from build123d import *

# Parameters (mm, degrees)
F1_DEPTH = 12.7
F2_DEPTH = 17.78


with BuildPart() as f1:
    # F0 (on Front) → F1 (new body)
    with BuildSketch(Plane.XZ):
        with BuildLine():
            ThreePointArc((-7.62, 17.4596133978), (-3.8920987123, 18.6481652613), (0, 19.05))
            Line((0, 19.05), (0, 25.4309050116))
            ThreePointArc((0, 25.4309050116), (-1.335031029, 25.3955492468), (-2.6663651194, 25.2901575092))
            Line((-2.6663651194, 25.2901575092), (-2.6663651194, 22.86))
            Line((-2.6663651194, 22.86), (-4.8713176481, 22.86))
            Line((-4.8713176481, 22.86), (-4.8713176481, 24.9589173434))
            ThreePointArc((-4.8713176481, 24.9589173434), (-6.2553989589, 24.6481649221), (-7.62, 24.260721841))
            Line((-7.62, 24.260721841), (-7.62, 17.4596133978))
        make_face()
        with BuildLine():
            ThreePointArc((-7.62, -17.4596133978), (-19.05, 0), (-7.62, 17.4596133978))
            Line((-7.62, 17.4596133978), (-7.62, 24.260721841))
            ThreePointArc((-7.62, 24.260721841), (-25.4254, 0), (-7.62, -24.260721841))
            Line((-7.62, -24.260721841), (-7.62, -17.4596133978))
        make_face()
        with BuildLine():
            ThreePointArc((-2.6663651194, 25.2901575092), (-1.335031029, 25.3955492468), (0, 25.4309050116))
            Line((0, 25.4309050116), (0, 33.02))
            Line((0, 33.02), (-7.62, 33.02))
            Line((-7.62, 33.02), (-7.62, 24.260721841))
            ThreePointArc((-7.62, 24.260721841), (-6.2553989589, 24.6481649221), (-4.8713176481, 24.9589173434))
            Line((-4.8713176481, 24.9589173434), (-4.8713176481, 29.7198501384))
            Line((-4.8713176481, 29.7198501384), (-2.6663651194, 29.7198501384))
            Line((-2.6663651194, 29.7198501384), (-2.6663651194, 25.2901575092))
        make_face()
        with BuildLine():
            ThreePointArc((0, -19.05), (-3.8920987123, -18.6481652613), (-7.62, -17.4596133978))
            Line((-7.62, -17.4596133978), (-7.62, -24.260721841))
            ThreePointArc((-7.62, -24.260721841), (-6.2553989589, -24.6481649221), (-4.8713176481, -24.9589173434))
            Line((-4.8713176481, -24.9589173434), (-4.8713176481, -22.86))
            Line((-4.8713176481, -22.86), (-2.6663651194, -22.86))
            Line((-2.6663651194, -22.86), (-2.6663651194, -25.2901575092))
            ThreePointArc((-2.6663651194, -25.2901575092), (-1.335031029, -25.3955492468), (0, -25.4309050116))
            Line((0, -25.4309050116), (0, -19.05))
        make_face()
        with BuildLine():
            ThreePointArc((-4.8713176481, -24.9589173434), (-6.2553989589, -24.6481649221), (-7.62, -24.260721841))
            Line((-7.62, -24.260721841), (-7.62, -33.02))
            Line((-7.62, -33.02), (0, -33.02))
            Line((0, -33.02), (0, -25.4309050116))
            ThreePointArc((0, -25.4309050116), (-1.335031029, -25.3955492468), (-2.6663651194, -25.2901575092))
            Line((-2.6663651194, -25.2901575092), (-2.6663651194, -29.7198501384))
            Line((-2.6663651194, -29.7198501384), (-4.8713176481, -29.7198501384))
            Line((-4.8713176481, -29.7198501384), (-4.8713176481, -24.9589173434))
        make_face()
    extrude(amount=F1_DEPTH)

    # F0 (on Front) → F2 (join)
    with BuildSketch(Plane.XZ):
        with BuildLine():
            ThreePointArc((-7.62, -17.4596133978), (-19.05, 0), (-7.62, 17.4596133978))
            Line((-7.62, 17.4596133978), (-7.62, 24.260721841))
            ThreePointArc((-7.62, 24.260721841), (-25.4254, 0), (-7.62, -24.260721841))
            Line((-7.62, -24.260721841), (-7.62, -17.4596133978))
        make_face()
    extrude(amount=F2_DEPTH)


solid = f1.part
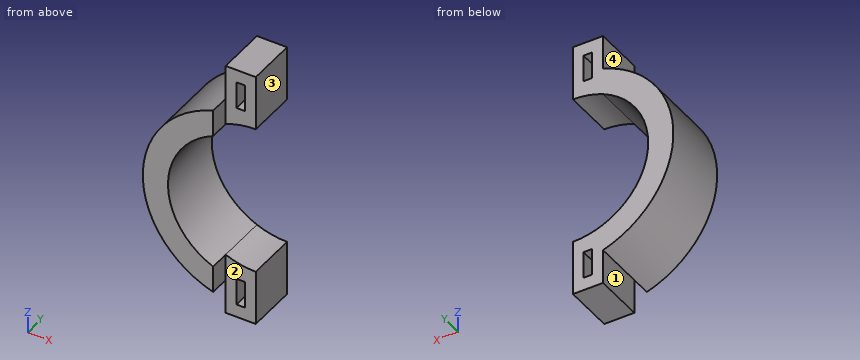
Check sheet for the modelled part. Datum: model origin and axes. Units: mm. Face numbers are marked on the shaded views. A direction names the side the tool comes from. Round coordinates to 2 decimals unless told otherwise and drop trailing zeros. Order: outer loops, then holes, each group sorted by start corner. A loop starts at its lowest first (then second) coordinate and runs counter-clockwise, first axis right, second up.
(1) Cross-section at A-A, the plane z = -26. Enter the section's corners in (x, y).
(2) Access from +Z, -Z, +X, -X, +Y, -Y to the whole of each face (thin tool, end or side, straight path). Record for the marked faces 1, 2, 3 and 4.
(3) Scan lines: probe 1 along X at (y, z) = (-5.25, -24.5); probe 2 along Z at (x, y) = (-3, -10.25); probe 3 along Z at (x, y) = (-13.25, -15.5). Record each from-to range of solid material in increasing order.
(4) Cross-section at D-D, the plane y = -14.75. Enter the section's corners in (x, z), and give its area (3 significant figures).
(5) Cross-section at B-B, the plane y = -4.75. Enter the section's corners in (x, z).
(6) Go/stop test with flat-tipped pins: P1, Ø3, axis at x = -16.5, y = -5.5, coming from the +Z side; P2, Ø2, axis at y = -12.5, z = -18.5, coming from the -X side; P3, Ø6, axis at x = -4.5, z = 21.5, coming from the -Y side; P4, Ø12, axis at x = -5, z = 24.5, coming from the +Y side. Record where each tip stops, or that it passes through.
(7) Cross-section at C-C, the plane x = -16.25. Enter the section's corners in (y, z).
Check sheet entries:
1. outline: (-7.62, -12.7) - (-4.87, -12.7) - (-4.87, 0) - (-7.62, 0) - close; (-2.67, -12.7) - (0, -12.7) - (0, 0) - (-2.67, 0) - close
2. face 1: -Z, -X, +Y, -Y
2. face 2: +Z, -Z, +X, -Y
2. face 3: +Z, -Z, +X, +Y, -Y
2. face 4: +Z, -X, +Y, -Y
3. probe 1: x = -7.62 to -4.87, -2.67 to 0
3. probe 2: z = -33.02 to -29.72, -22.86 to -18.81, 18.81 to 22.86, 29.72 to 33.02
3. probe 3: z = -21.7 to -13.69, 13.69 to 21.7
4. outline: (-7.62, -24.26) - (-7.62, -17.46) arc R19.05 cw to (-7.62, 17.46) - (-7.62, 24.26) arc R25.43 ccw to start
4. area: 346 mm2
5. outline: (-7.62, -33.02) - (0, -33.02) - (0, -19.05) arc R19.05 cw to (0, 19.05) - (0, 33.02) - (-7.62, 33.02) - (-7.62, 24.26) arc R25.43 ccw to (-7.62, -24.26) - close; hole (-4.87, -29.72) - (-2.67, -29.72) - (-2.67, -22.86) - (-4.87, -22.86) - close; hole (-4.87, 22.86) - (-2.67, 22.86) - (-2.67, 29.72) - (-4.87, 29.72) - close
6. P1: stops at z = 20.53
6. P2: stops at x = -18.45
6. P3: stops at y = -12.7
6. P4: stops at y = 0
7. outline: (-17.78, -19.56) - (0, -19.56) - (0, -9.94) - (-17.78, -9.94) - close; (-17.78, 9.94) - (0, 9.94) - (0, 19.56) - (-17.78, 19.56) - close
